Autodesk Inventor part; units mm, degrees
ref_plane "YZ Plane" through (0, 0, 0) normal (1, 0, 0) x (0, 1, 0)
ref_plane "XZ Plane" through (0, 0, 0) normal (0, 1, 0) x (-1, 0, 0)
ref_plane "XY Plane" through (0, 0, 0) normal (0, 0, 1) x (1, 0, 0)
sketch "Sketch1" plane through (0, 0, 0) normal (0, 0, 1) x (1, 0, 0)
  line L0 (-170, 20) -> (-77.5, 20)
  line L1 (170, 45) -> (170, 35)
  line L2 (-77.5, -20) -> (-170, -20)
  line L3 (-170, -20) -> (-170, 20)
  line L4 (-77.5, 65) -> (77.5, 65)
  line L5 (77.5, -65) -> (-77.5, -65)
  line L6 (170, 50) -> (77.5, 50)
  line L7 (77.5, -50) -> (170, -50)
  line L8 (170, -50) -> (170, 50)
  line L9 (-77.5, -65) -> (-77.5, -20)
  line L10 (-77.5, 20) -> (-77.5, 65)
  line L11 (-77.5, -20) -> (-77.5, -63.8623)
  line L12 (-170, 0) -> (170, 0) construction
  line L13 (77.5, -50) -> (77.5, -65)
  line L14 (77.5, 65) -> (77.5, 50)
  line L15 (62.5, 35) -> (155, 35)
  line L16 (155, 35) -> (155, -35)
  line L17 (155, -35) -> (62.5, -35)
  line L18 (62.5, -35) -> (62.5, -50)
  line L19 (62.5, -50) -> (-62.5, -50)
  line L20 (-62.5, -50) -> (-62.5, -5)
  line L21 (-62.5, -5) -> (-62.5, 50)
  line L22 (-62.5, 50) -> (62.5, 50)
  line L23 (62.5, 50) -> (62.5, 35)
  line L24 (0, 50) -> (0, -50) construction
  point P0 (0, 0)
  point P1 (170, 5)
  point P2 (170, -5)
  dimension "d2" = 155
  dimension "d3" = 130
  dimension "d21" = 92.5
  dimension "d22" = 100
  dimension "d23" = 40
  dimension "d25" = 92.5
  dimension "d29" = 15
extrude "Extrusion1" add sketch "Sketch1" along normal mid plane 90 contours L0 L10 L4 L14 L6 L8 L1 L7 L13 L5 L9 L2 L3 | L15 L16 L17 L18 L19 L20 L21 L22 L23
sketch "Sketch2" plane through (0, 0, 0) normal (0, 1, 0) x (-1, 0, 0)
  circle A0 centre (-123.75, 0) radius 45
  circle A1 centre (123.75, 0) radius 45
  line L0 (0, 43.1567) -> (0, -43.1567) construction
  line L1 (170.8168, 0) -> (-169.1832, 0) construction
  line L2 (170.8168, 0) -> (-169.1832, 0) construction
  line L3 (170, -45) -> (170, 45) construction
  line L4 (77.5, -45) -> (170, -45) construction
  line L5 (123.75, -45) -> (123.75, 45) construction
  line L6 (170, 45) -> (77.5, 45) construction
  line L7 (-123.75, -45) -> (-123.75, 45) construction
  point P0 (0, 0)
  point P1 (0.8168, 0)
  point P2 (0, 0)
  dimension "d7" = 90
extrude "Extrusion2" add sketch "Sketch2" against normal blind 32 from surface at -50 contours A0
extrude "Extrusion3" add sketch "Sketch2" against normal blind 32 from surface at -20 contours A1
fillet "Fillet1" radius 15 2 edges at (-77.5, 65, 0) (-77.5, -65, 0)
mirror "Mirror1" about plane through (0, 0, 0) normal (0, 1, 0) of "Extrusion3", "Extrusion2"
extrude "Extrusion4" cut sketch "Sketch1" against normal mid plane 55 contours L15 L16 L17 L18 L19 L20 L21 L22 L23
Read the model definition and answer for the solid it produces. Units are mm, in the model's axes. A direction names the side the tool comes from. Round coordinates to 2 decimals unless told otherwise and drop trailing zeros. Loops run counter-clockwise (first coordinate to the right, second up) from the corner with the lowest first, then second, coordinate; pieces in that order, holes last. Notation, with made-up numbers: (80, 88.25) - (97, 88.25) arc R20 cw to (97, 116.25) - close; hole circle Ø2 at (-19.75, 78). An arc over 180 degrees is marked (long way). One line per question, with ' | ' between items. Start each with the question number.
Q1. Section D-D on x = -110 is taken. Give the vertices of the cut face in (y, z).
Q2. For faces 5 (the flat face through (62.5, 43, 0)), 6 (the flat face through (78, 50, -4)), 7 (the flat face through (77.5, 58, -1)), determine the directions among +Z, -Z, +X, -X, +Y, -Y from which every point of the face is accessible in a straight line to the end or side of a thin tool.
Q3. For a pull along X with two mould halves and no side action, classify faces 1 (the flat face through (-78, -20, -7)), 2 (the flat face through (109, -35, 0)), 3 (the flat face through (170, -1, -1)), 4 (the flat face through (-124, 52, 1)) as +X half, -X half, draft (parallel to the pull), parting line (faces both ways), or undercut.
Q4. Section A-A on y = 4 is taken. Give the vertices of the cut face in (x, z).
Q5. Section B-B on x = 49 is taken. Give the vertices of the cut face in (y, z).
Q6. Flat-ended cylindrical pins translate along their axes: pin 1 (7.5 mm diameter, centred on y = -59, z = 12.5, fed in from +X); pin 2 (23 mm diameter, centred on x = -98, z = -4, fed in from +Y); pin 3 (1 mm diameter, centred on y = 24, z = -22.5, fed in from -X). Find the tip coordinate at first contact, or state that the pin passes through.
Q7. Find the intervals of material crossed by L1, parallel to Y at x = -20.5, z = -1; L2, parallel to Y at x = 69.5, z = -13; L3, parallel to Z at x = 64, y = 10.5, in increasing order.
Established:
1) outline: (-52, -42.85) - (-20, -42.85) - (-20, -45) - (20, -45) - (20, -42.85) - (52, -42.85) - (52, 42.85) - (20, 42.85) - (20, 45) - (-20, 45) - (-20, 42.85) - (-52, 42.85) - close
2) face 5: none | face 6: +Y | face 7: +Z, -Z, +Y
3) face 1: undercut | face 2: undercut | face 3: +X half | face 4: draft
4) outline: (-170, -45) - (170, -45) - (170, 45) - (-170, 45) - close; hole (-62.5, -27.5) - (155, -27.5) - (155, 27.5) - (-62.5, 27.5) - close
5) outline: (-65, -45) - (65, -45) - (65, 45) - (-65, 45) - close; hole (-50, -27.5) - (50, -27.5) - (50, 27.5) - (-50, 27.5) - close
6) pin 1: x = 167.89 | pin 2: y = 52 | pin 3: x = -163.01
7) L1: -65 to -50, 50 to 65 | L2: -65 to -35, 35 to 65 | L3: -45 to -27.5, 27.5 to 45
